```python
from build123d import *

# Parameters (mm, degrees)
BOSS_EXTRUDE1_DEPTH = 12
CHAMFER1_SIZE       = 12
SKETCH2_R           = 4
SKETCH2_R_2         = 10
CUT_EXTRUDE1_DEPTH  = 609.394608786


with BuildPart() as part:
    # Sketch1 → Boss-Extrude1 (new body)
    with BuildSketch(Plane.XY):
        with BuildLine():
            Line((0, 0), (0, -10))
            Line((0, -10), (40, -10))
            ThreePointArc((40, -10), (48.819660113, -2.639320225), (60, 0))
            Line((60, 0), (165, 0))
            ThreePointArc((165, 0), (176.180339887, -2.639320225), (185, -10))
            Line((185, -10), (415, -10))
            ThreePointArc((415, -10), (423.819660113, -2.639320225), (435, 0))
            Line((435, 0), (540, 0))
            ThreePointArc((540, 0), (551.180339887, -2.639320225), (560, -10))
            Line((560, -10), (600, -10))
            Line((600, -10), (600, 0))
            Line((600, 0), (600, 100))
            Line((600, 100), (0, 100))
            Line((0, 100), (0, 0))
        make_face()
    extrude(amount=BOSS_EXTRUDE1_DEPTH)

    # Chamfer1
    chamfer1_edges = [part.edges().sort_by_distance(p)[0] for p in [
        (300, 100, 12),
        (600, 45, 12),
        (0, 45, 12),
    ]]
    chamfer(chamfer1_edges, length=CHAMFER1_SIZE - 0.0001)  # a hair under: the kernel refuses the full size

    # Sketch2 → Cut-Extrude1 (cut, through all)
    with BuildSketch(Plane(origin=(0, 0, 0), x_dir=(-1, 0, 0), z_dir=(0, 0, -1))):
        with Locations((-335, 65)):
            Circle(SKETCH2_R)
        with Locations((-300, 45)):
            Circle(SKETCH2_R_2)
        with Locations((-265, 25)):
            Circle(SKETCH2_R)
    extrude(amount=-CUT_EXTRUDE1_DEPTH, mode=Mode.SUBTRACT)


solid = part.part
```
Source: CAD feature listing. Evaluate the final solid. Frame: model axes, mm. A direction names the side the tool comes from. Coordinates: 2 decimals unless noted, no trailing zeros. Order: outer loops, then holes, each group sorted by start corner. A loop starts at its lowest first (then second) coordinate and runs counter-clockwise, first axis right, second up. Notation, with made-up numbers: (86, 4) - (107, 4) arc R23 ccw to (107, 33) - close; hole circle Ø8 at (65.25, -39). An arc over 180 degrees is marked (long way). One line per item, written item: value.
1) Cut plane B-B on z = 7.5. Output: boundary loops of the cut face in (x, y), plus the area to 3 significant figures.
Computed values:
outline: (7.5, -10) - (40, -10) arc R25 cw to (60, 0) - (165, 0) arc R25 cw to (185, -10) - (415, -10) arc R25 cw to (435, 0) - (540, 0) arc R25 cw to (560, -10) - (592.5, -10) - (592.5, 92.5) - (7.5, 92.5) - close; hole circle Ø8 at (265, 25); hole circle Ø20 at (300, 45); hole circle Ø8 at (335, 65)
area: 56,900 mm^2
2) Mould query, pull axis X, two halves, no side actions, for faces 3 (the face through (423.7, -2.7, 5.9)), 4 (the face through (6, 46, 6)), 5 (the face through (48.7, -2.7, 5.9)), 6 (the face through (298, -10, 6)). Classes: released by +X, released by -X, zero draft, split by the parting line, or undercut.
Computed values:
face 3: undercut
face 4: released by -X
face 5: undercut
face 6: zero draft
3) Ray query, line 1 (Y direction, x = 335, z = 8.75); line 2 (Y direction, x = 335, z = 6.5); line 3 (X direction, y = 22, z = 0.5). Return the intervals inside material, ascending. Write a range as [from, to].
Computed values:
line 1: y = [-10, 61], [69, 91.25]
line 2: y = [-10, 61], [69, 93.5]
line 3: x = [0.5, 262.35], [267.65, 599.5]
4) Reachability of faces 1 (the face through (176.035, -2.567, 5.916)), 2 (the face through (296, 58, 0)) from +Z, -Z, +X, -X, +Y, -Y: full face, straight path, thin tool, end or side. Return the list, or none.
Computed values:
face 1: +Z, -Z, -Y
face 2: -Z, +X, -X, +Y, -Y
5) Contact query for flat-ended pins moving along their axis: pin 1 (5 mm diameter, centred on x = 243.5, z = 3, fed in from +Y); pin 2 (2 mm diameter, centred on x = 144.5, z = 2, fed in from +Y); pin 3 (16 mm diameter, centred on x = 300, y = 45, fed in from +Z); pin 4 (6 mm diameter, centred on y = 77.5, z = 9, fed in from +X). Output: stop coordinate, or through.
Computed values:
pin 1: stops at y = 99.5
pin 2: stops at y = 99
pin 3: passes through
pin 4: stops at x = 594
